```python
from build123d import *

# Parameters (mm, degrees)
SKETCH1_W                      = 150
SKETCH1_H                      = 70
BOSS_EXTRUDE1_DEPTH            = 32
SKETCH2_R                      = 9.5
LINEAR_BEARING_CUT_1_DEPTH     = 55
Y_AXIS_SHAFTS_CUT_DEPTH        = 169.594187326
LINEAR_BEARING_CUT_2_START     = -55
SKETCH7_R                      = 9.5
LINEAR_BEARING_CUT_2_DEPTH     = 55
SKETCH6_R                      = 6
BETWEEN_BEARINGS_DEPTH         = 123.266103234
SKETCH8_R                      = 3.5
SHAFT_HOLDER_SCREW_CUT_DEPTH   = 4
SKETCH9_R                      = 1.25
SHAFT_HOLDER_SCREW_CUT2_DEPTH  = 20
SHAFT_HOLDER_SCREW_CUT_3_START = -2
SKETCH10_R                     = 3.5
SHAFT_HOLDER_SCREW_CUT_3_DEPTH = 2
SHAFT_HOLDER_SCREW_CUT_4_START = -20
SKETCH11_R                     = 1.25
SHAFT_HOLDER_SCREW_CUT_4_DEPTH = 20
SKETCH12_R                     = 1.8
LINEAR_BEARING_SREW1_DEPTH     = 14
SKETCH13_R                     = 1.85
LINEAR_BEARING_SCREW2_DEPTH    = 14


with BuildPart() as part:
    # Sketch1 → Boss-Extrude1 (new body)
    with BuildSketch(Plane.XY):
        with Locations((-75, -35)):
            Rectangle(SKETCH1_W, SKETCH1_H)
    extrude(amount=BOSS_EXTRUDE1_DEPTH)

    # Sketch2 → Linear_bearing-cut-1 (cut)
    with BuildSketch(Plane.ZY.offset(150)):
        with Locations((16, -35)):
            Circle(SKETCH2_R)
    extrude(amount=-LINEAR_BEARING_CUT_1_DEPTH, mode=Mode.SUBTRACT)

    # Sketch5 → Y-axis-shafts-cut (cut, through all)
    with BuildSketch(Plane.XY.offset(32)):
        with BuildLine():
            Line((-141.5, 0), (-141.5, -7.5))
            ThreePointArc((-141.5, -7.5), (-141, -17.524937811), (-140.5, -7.5))
            Line((-140.5, -7.5), (-140.5, 0))
            Line((-140.5, 0), (-141.5, 0))
        make_face()
        with BuildLine():
            Line((-8.5, 0), (-8.5, -7.5))
            ThreePointArc((-8.5, -7.5), (-9, -17.524937811), (-9.5, -7.5))
            Line((-9.5, -7.5), (-9.5, 0))
            Line((-9.5, 0), (-8.5, 0))
        make_face()
        with BuildLine():
            Line((-141.5, -70), (-141.5, -62.5))
            ThreePointArc((-141.5, -62.5), (-141, -52.475062189), (-140.5, -62.5))
            Line((-140.5, -62.5), (-140.5, -70))
            Line((-140.5, -70), (-141.5, -70))
        make_face()
        with BuildLine():
            Line((-9.5, -70), (-9.5, -62.5))
            ThreePointArc((-9.5, -62.5), (-9, -52.475062189), (-8.5, -62.5))
            Line((-8.5, -62.5), (-8.5, -70))
            Line((-8.5, -70), (-9.5, -70))
        make_face()
    extrude(amount=-Y_AXIS_SHAFTS_CUT_DEPTH, mode=Mode.SUBTRACT)

    # Sketch7 → Linear-bearing-cut-2 (cut)
    with BuildSketch(Plane(origin=(0, 0, 0), x_dir=(0, 0, -1), z_dir=(1, 0, 0)).offset(LINEAR_BEARING_CUT_2_START)):
        with Locations(Location((-16, -35, 0), (0, 0, 180))):
            Circle(SKETCH7_R)
    extrude(amount=LINEAR_BEARING_CUT_2_DEPTH, mode=Mode.SUBTRACT)

    # Sketch6 → between-bearings (cut, through all)
    with BuildSketch(Plane.ZY.offset(95)):
        with Locations((16, -35)):
            Circle(SKETCH6_R)
    extrude(amount=-BETWEEN_BEARINGS_DEPTH, mode=Mode.SUBTRACT)

    # Sketch8 → shaft-holder-screw-cut (cut)
    with BuildSketch(Plane.ZY.offset(150)):
        with Locations((5, -6)):
            Circle(SKETCH8_R)
        with Locations(Location((27, -6, 0), (0, 0, 180))):
            Circle(SKETCH8_R)
        with Locations((27, -64)):
            Circle(SKETCH8_R)
        with Locations(Location((5, -64, 0), (0, 0, 180))):
            Circle(SKETCH8_R)
    extrude(amount=-SHAFT_HOLDER_SCREW_CUT_DEPTH, mode=Mode.SUBTRACT)

    # Sketch9 → shaft-holder-screw-cut2 (cut)
    with BuildSketch(Plane.ZY.offset(146)):
        with Locations((5, -6)):
            Circle(SKETCH9_R)
        with Locations((27, -6)):
            Circle(SKETCH9_R)
        with Locations((5, -64)):
            Circle(SKETCH9_R)
        with Locations((27, -64)):
            Circle(SKETCH9_R)
    extrude(amount=-SHAFT_HOLDER_SCREW_CUT2_DEPTH, mode=Mode.SUBTRACT)

    # Sketch10 → shaft-holder-screw-cut-3 (cut)
    with BuildSketch(Plane(origin=(0, 0, 0), x_dir=(0, 0, -1), z_dir=(1, 0, 0)).offset(SHAFT_HOLDER_SCREW_CUT_3_START)):
        with Locations((-27, -6)):
            Circle(SKETCH10_R)
        with Locations(Location((-5, -6, 0), (0, 0, 180))):
            Circle(SKETCH10_R)
        with Locations((-5, -64)):
            Circle(SKETCH10_R)
        with Locations(Location((-27, -64, 0), (0, 0, 180))):
            Circle(SKETCH10_R)
    extrude(amount=SHAFT_HOLDER_SCREW_CUT_3_DEPTH, mode=Mode.SUBTRACT)

    # Sketch11 → shaft-holder-screw-cut-4 (cut)
    with BuildSketch(Plane(origin=(-2, 0, 0), x_dir=(0, 0, -1), z_dir=(1, 0, 0)).offset(SHAFT_HOLDER_SCREW_CUT_4_START)):
        with Locations(Location((-27, -6, 0), (0, 0, 180))):
            Circle(SKETCH11_R)
        with Locations(Location((-5, -6, 0), (0, 0, 180))):
            Circle(SKETCH11_R)
        with Locations(Location((-5, -64, 0), (0, 0, 180))):
            Circle(SKETCH11_R)
        with Locations(Location((-27, -64, 0), (0, 0, 180))):
            Circle(SKETCH11_R)
    extrude(amount=SHAFT_HOLDER_SCREW_CUT_4_DEPTH, mode=Mode.SUBTRACT)

    # Sketch12 → Linear-bearing-srew1 (cut)
    with BuildSketch(Plane(origin=(0, 0, 0), x_dir=(0, 0, -1), z_dir=(1, 0, 0))):
        with Locations(Location((-5.75, -24.75, 0), (0, 0, 90))):
            Circle(SKETCH12_R)
        with Locations(Location((-26.25, -24.75, 0), (0, 0, 270))):
            Circle(SKETCH12_R)
        with Locations(Location((-5.75, -45.25, 0), (0, 0, 270))):
            Circle(SKETCH12_R)
        with Locations(Location((-26.25, -45.25, 0), (0, 0, 90))):
            Circle(SKETCH12_R)
    extrude(amount=-LINEAR_BEARING_SREW1_DEPTH, mode=Mode.SUBTRACT)

    # Sketch13 → Linear-bearing-screw2 (cut)
    with BuildSketch(Plane.ZY.offset(150)):
        with Locations(Location((27.5, -24.75, 0), (0, 0, 270))):
            Circle(SKETCH13_R)
        with Locations(Location((4.5, -24.75, 0), (0, 0, 90))):
            Circle(SKETCH13_R)
        with Locations(Location((27.5, -45.25, 0), (0, 0, 90))):
            Circle(SKETCH13_R)
        with Locations(Location((4.5, -45.25, 0), (0, 0, 270))):
            Circle(SKETCH13_R)
    extrude(amount=-LINEAR_BEARING_SCREW2_DEPTH, mode=Mode.SUBTRACT)


solid = part.part
```
Geometry: final body of the model. Coordinates: model frame, mm. A direction names the side the tool comes from. Coordinates: 2 decimals unless noted, no trailing zeros. Loops run counter-clockwise (first coordinate to the right, second up) from the corner with the lowest first, then second, coordinate; pieces in that order, holes last. Notation, with made-up numbers: (82.25, -29.5) -> (90.25, -29.5) arc R22 cw to (90.25, -9.5) -> close; hole circle Ø2 at (22, 46.25). An arc over 180 degrees is marked (long way). Use a Markdown table: item, result. Add a question column.
(1) Line query: line 1 along X through (y, z) = (-65, 20.5); line 2 along Y through (x, z) = (-148, 27); line 3 along Y through (x, z) = (-101.5, 16). Output: solid intervals per line, ascending.
(2) Access query for faces 5 (the flat face through (-140.5, -66, 16)), 6 (the flat face through (-76, -35, 32)), 7 (the flat face through (-141.5, -4, 16)), 8 (the flat face through (-14, -45, 26)), 9 (the cylindrical face through (-148.028, -7.341, 8.233)). Directions: +Z, -Z, +X, -X, +Y, -Y. A direction counts if a zero-diameter tool reaches every point of the face in a straight line with its end or side. Return the directions, or none.
(3) Pin query (flat end, axial travel): pin 1 Ø3 at (y, z) = (-31.5, 9) entering from -X; pin 2 Ø2 at (y, z) = (-62.5, 4) entering from -X; pin 3 Ø8 at (x, y) = (-9, -57.5) entering from -Z; pin 4 Ø2 at (y, z) = (-6, 5) entering from +X. Return the tip coordinate at first contact, or that it passes through.
(4) Mould query, pull axis X, two halves, no side actions, for faces 1 (the flat face through (-136, -45, 27)), 2 (the cylindrical face through (-143.098, -46.614, 26.25)), 3 (the flat face through (-140.5, -4, 16)), 4 (the flat face through (-14, -25, 6)). Classes: pulls with the +X half, pulls with the -X half, needs draft (parallel to the pull), parting line crosses it, or undercut.
(5) Section query A-A, the plane y = -57.5. Return loops of the section in (x, z), plus the area to 3 significant figures.
(6) Section query C-C, the plane x = -121.5. Return loops of the section in (y, z).
Answer:
| question | item | result |
|---|---|---|
| 1 | line 1 | x = -150 to -141.5, -140.5 to -9.5, -8.5 to 0 |
| 1 | line 2 | y = -70 to -67.5, -60.5 to -47.03, -43.47 to -26.53, -22.97 to -9.5, -2.5 to 0 |
| 1 | line 3 | y = -70 to -44.5, -25.5 to 0 |
| 2 | face 5 | +Z, -Z, -Y |
| 2 | face 6 | +Z, +X, -X, +Y, -Y |
| 2 | face 7 | +Z, -Z, +Y |
| 2 | face 8 | +X |
| 2 | face 9 | -X |
| 3 | pin 1 | stops at x = -95 |
| 3 | pin 2 | stops at x = -146 |
| 3 | pin 3 | passes through |
| 3 | pin 4 | stops at x = -22 |
| 4 | face 1 | pulls with the -X half |
| 4 | face 2 | needs draft |
| 4 | face 3 | undercut |
| 4 | face 4 | pulls with the +X half |
| 5 | outline | (-150, 0) -> (-146.02, 0) -> (-146.02, 32) -> (-150, 32) -> close; (-135.98, 0) -> (-14.02, 0) -> (-14.02, 32) -> (-135.98, 32) -> close; (-3.98, 0) -> (0, 0) -> (0, 32) -> (-3.98, 32) -> close |
| 5 | area | 4,160 mm^2 |
| 6 | outline | (-70, 0) -> (0, 0) -> (0, 32) -> (-70, 32) -> close; hole circle Ø19 at (-35, 16) |
